Could you check a few things on this model? Use its own coordinates, in mm. Face numbers are marked on the shaded views. Round coordinates to 2 decimals unless told otherwise and drop trailing zeros. Write each loop counter-clockwise with the first axis right and the second up, starting at its lowest first coordinate (ties: lowest second). Pieces come first, ordered by that corner, then holes.
```python
from build123d import *

# Parameters (mm, degrees)
SKETCH1_R           = 55
BOSS_EXTRUDE1_DEPTH = 54.8
SHELL1_T            = -5
SKETCH2_R           = 35
CUT_EXTRUDE1_DEPTH  = 6
SKETCH3_R           = 42
CUT_EXTRUDE2_DEPTH  = 55.8
SKETCH4_R           = 4.15
CUT_EXTRUDE3_DEPTH  = 55.8
SKETCH6_R           = 50
CUT_EXTRUDE4_DEPTH  = 2
CUT_EXTRUDE5_DEPTH  = 4
FILLET1_R           = 10
SKETCH8_OUTSIDE_W   = 144.986
SKETCH8_OUTSIDE_H   = 144.986
SKETCH8_OUTSIDE_R   = 52.35
CUT_EXTRUDE6_DEPTH  = 4.8
CHAMFER1_SIZE       = 2
CHAMFER1_SIZE2      = 1.154700538
SKETCH9_R           = 52.5
CUT_EXTRUDE7_DEPTH  = 5


with BuildPart() as part:
    # Sketch1 → Boss-Extrude1 (new body)
    with BuildSketch(Plane(origin=(0, 0, 0), x_dir=(1, 0, 0), z_dir=(0, 1, 0))):
        with Locations(Location((0, 0, 0), (0, 0, 270))):  # turned: the seam where the file's is
            Circle(SKETCH1_R)
    extrude(amount=BOSS_EXTRUDE1_DEPTH)

    # Shell1
    shell1_openings = [part.faces().sort_by_distance(p)[0] for p in [
        (0, 0, 0),
    ]]
    offset(amount=SHELL1_T, openings=shell1_openings, kind=Kind.INTERSECTION)

    # Sketch2 → Cut-Extrude1 (cut, through all)
    with BuildSketch(Plane.XZ.offset(-49.8)):
        with Locations(Location((0, 0, 0), (0, 0, 270))):  # turned: the seam where the file's is
            Circle(SKETCH2_R)
    extrude(amount=-CUT_EXTRUDE1_DEPTH, mode=Mode.SUBTRACT)

    # Sketch3 → Cut-Extrude2 (cut, through all)
    with BuildSketch(Plane(origin=(0, 54.8, 0), x_dir=(1, 0, 0), z_dir=(0, 1, 0))):
        with Locations(Location((0, 0, 0), (0, 0, 270))):  # turned: the seam where the file's is
            Circle(SKETCH3_R)
    extrude(amount=-CUT_EXTRUDE2_DEPTH, mode=Mode.SUBTRACT)

    # Sketch4 → Cut-Extrude3 (cut, through all)
    with BuildSketch(Plane(origin=(0, 54.8, 0), x_dir=(1, 0, 0), z_dir=(0, 1, 0))):
        with Locations(Location((-33.234018716, -33.234018716, 0), (0, 0, 270))):  # turned: the seam where the file's is
            Circle(SKETCH4_R)
        with Locations(Location((-33.234018716, 33.234018716, 0), (0, 0, 270))):  # turned: the seam where the file's is
            Circle(SKETCH4_R)
        with Locations(Location((33.234018716, 33.234018716, 0), (0, 0, 270))):  # turned: the seam where the file's is
            Circle(SKETCH4_R)
        with Locations(Location((33.234018716, -33.234018716, 0), (0, 0, 270))):  # turned: the seam where the file's is
            Circle(SKETCH4_R)
    extrude(amount=-CUT_EXTRUDE3_DEPTH, mode=Mode.SUBTRACT)

    # Sketch6 → Cut-Extrude4 (cut)
    with BuildSketch(Plane.XZ.offset(-49.8)):
        Circle(SKETCH6_R)
    extrude(amount=-CUT_EXTRUDE4_DEPTH, mode=Mode.SUBTRACT)

    # Sketch7 → Cut-Extrude5 (cut, through all)
    with BuildSketch(Plane.XZ.offset(-51.8)):
        with BuildLine():
            Line((15, 33.234018716), (15, 47.696960071))
            ThreePointArc((15, 47.696960071), (0, 50), (-15, 47.696960071))
            Line((-15, 47.696960071), (-15, 33.234018716))
            Line((-15, 33.234018716), (15, 33.234018716))
        make_face()
    extrude(amount=-CUT_EXTRUDE5_DEPTH, mode=Mode.SUBTRACT)

    # Fillet1
    fillet1_edges = [part.edges().sort_by_distance(p)[0] for p in [
        (-15, 53.3, 39.230090492),
        (15, 53.3, 39.230090492),
    ]]
    fillet(fillet1_edges, radius=FILLET1_R)

    # Sketch8 outside → Cut-Extrude6 (cut)
    with BuildSketch(Plane(origin=(0, 54.8, 0), x_dir=(1, 0, 0), z_dir=(0, 1, 0))):
        Rectangle(SKETCH8_OUTSIDE_W, SKETCH8_OUTSIDE_H)
        with Locations(Location((0, 0, 0), (0, 0, 270))):  # turned: the seam where the file's is
            Circle(SKETCH8_OUTSIDE_R, mode=Mode.SUBTRACT)
    extrude(amount=-CUT_EXTRUDE6_DEPTH, mode=Mode.SUBTRACT)

    # Chamfer1
    chamfer1_edges = [part.edges().sort_by_distance(p)[0] for p in [
        (0, 54.8, -52.35),
    ]]
    chamfer1_side = [part.faces().sort_by_distance(p)[0] for p in [
        (0, 52.4, -52.35),
    ]]
    chamfer(chamfer1_edges, length=CHAMFER1_SIZE, length2=CHAMFER1_SIZE2, reference=chamfer1_side[0])

    # Sketch9 → Cut-Extrude7 (cut)
    with BuildSketch(Plane.XZ):
        with Locations(Location((0, 0, 0), (0, 0, 270))):  # turned: the seam where the file's is
            Circle(SKETCH9_R)
    extrude(amount=-CUT_EXTRUDE7_DEPTH, mode=Mode.SUBTRACT)


solid = part.part
```
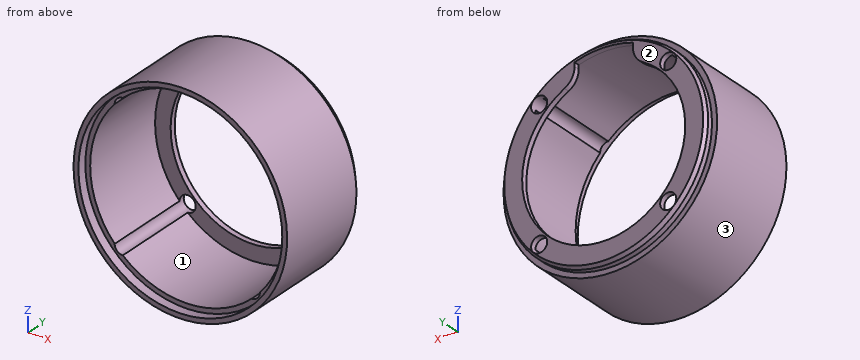
Q1. We'd pull the mould along X, two halves only. Please class the marked faces 1, 2 and 3: pulls with the +X half, pulls with the -X half, needs draft (parallel to the pull), parting line crosses it, or undercut.
Q2. Imagine slicing it at D-D, the plane z = -36. Count the separate pieces of the cut face and the enclosed holes in it, then the cut area to 3 significant figures.
Q3. Imagine slicing it at A-A, the plane z = 0. Write out the boundary of the cut face in (x, y).
Q4. I'm going to push flat-ended pins straight in: pin 1 Ø3 at (y, z) = (47.5, -1.5) entering from -X; pin 2 Ø4 at (y, z) = (7, -26) entering from +X; pin 3 Ø5 at (x, y) = (-32, 11.5) entering from -Z; pin 4 Ø6.5 at (x, z) = (33.23, -33.23) entering from -Y. Where does each tip first touch, or does it pass through?
Q5. If I drill on L1, parallel to X at y = 1.75, z = 0; L2, parallel to X at y = 51, z = -30; L3, parallel to Z at x = 15.5, y = 38, over which ranges is the centre line in solid material (lowest first)?
Q6. Imagine slicing it at B-B, the plane x = 0. Write out the boundary of the cut face in (y, z), then the cut area to 3 significant figures.
Q7. Imagine slicing it at C-C, the plane y = 29. Write out the boundary of the cut face in (x, z), then the cut area to 3 significant figures.
Results found:
1. face 1: undercut
1. face 2: needs draft
1. face 3: parting line crosses it
2. separate pieces: 4
2. enclosed holes: 0
2. area: 570 mm2
3. outline: (-55, 0) - (-52.5, 0) - (-52.5, 5) - (-50, 5) - (-50, 51.8) - (-42, 51.8) - (-42, 54.8) - (-51.2, 54.8) - (-52.35, 52.8) - (-52.35, 50) - (-55, 50) - close; (42, 51.8) - (50, 51.8) - (50, 5) - (52.5, 5) - (52.5, 0) - (55, 0) - (55, 50) - (52.35, 50) - (52.35, 52.8) - (51.2, 54.8) - (42, 54.8) - close
4. pin 1: stops at x = -55
4. pin 2: stops at x = 49.49
4. pin 3: stops at z = -46.42
4. pin 4: passes through
5. L1: x = -55 to -52.5, 52.5 to 55
5. L2: x = -42.9 to -40, 40 to 42.9
5. L3: z = -52.77 to -47.54, 47.54 to 52.77
6. outline: (0, -55) - (50, -55) - (50, -52.35) - (52.8, -52.35) - (54.8, -51.2) - (54.8, -42) - (51.8, -42) - (51.8, -50) - (5, -50) - (5, -52.5) - (0, -52.5) - close; (0, 52.5) - (5, 52.5) - (5, 50) - (54.8, 50) - (54.8, 51.2) - (52.8, 52.35) - (50, 52.35) - (50, 55) - (0, 55) - close
6. area: 519 mm2
7. outline: circle Ø110 at (0, 0); hole (-37.38, -33.2) arc R4.15 ccw to (-33.2, -37.38) arc R50 ccw to (33.2, -37.38) arc R4.15 ccw to (37.38, -33.2) arc R50 ccw to (37.38, 33.2) arc R4.15 ccw to (33.2, 37.38) arc R50 ccw to (-33.2, 37.38) arc R4.15 ccw to (-37.38, 33.2) arc R50 ccw to start
7. area: 1,630 mm2
